Work out the finished part from the listing and answer in its coordinate system (mm). A direction names the side the tool comes from. Give positions to 0.01 mm unless a question says otherwise; leave off trailing zeros. Order: outer loops, then holes, each group sorted by start corner. A loop starts at its lowest first (then second) coordinate and runs counter-clockwise, first axis right, second up.
```python
from build123d import *

# Parameters (mm, degrees)
SKETCH1_W           = 111
SKETCH1_H           = 195
BOSS_EXTRUDE3_DEPTH = 30
SKETCH12_W          = 107
SKETCH12_H          = 191
CUT_EXTRUDE14_DEPTH = 28
SKETCH13_W          = 193
SKETCH13_H          = 26
CUT_EXTRUDE15_DEPTH = 112
CUT_EXTRUDE18_DEPTH = 28
CUT_EXTRUDE20_DEPTH = 28
FILLET1_R           = 2


with BuildPart() as part:
    # Sketch1 → Boss-Extrude3 (new body)
    with BuildSketch(Plane(origin=(0, 0, 0), x_dir=(1, 0, 0), z_dir=(0, 1, 0))):
        with Locations((55.5, 97.5)):
            Rectangle(SKETCH1_W, SKETCH1_H)
    extrude(amount=BOSS_EXTRUDE3_DEPTH)

    # Sketch12 → Cut-Extrude14 (cut)
    with BuildSketch(Plane.XZ):
        with Locations((55.5, -97.5)):
            Rectangle(SKETCH12_W, SKETCH12_H)
    extrude(amount=-CUT_EXTRUDE14_DEPTH, mode=Mode.SUBTRACT)

    # Sketch13 → Cut-Extrude15 (cut, through all)
    with BuildSketch(Plane(origin=(111, 0, 0), x_dir=(0, 0, -1), z_dir=(1, 0, 0))):
        with Locations((98.5, 13)):
            Rectangle(SKETCH13_W, SKETCH13_H)
    extrude(amount=-CUT_EXTRUDE15_DEPTH, mode=Mode.SUBTRACT)

    # Sketch14 → Cut-Extrude18 (cut)
    with BuildSketch(Plane(origin=(0, 30, 0), x_dir=(1, 0, 0), z_dir=(0, 1, 0))):
        with BuildLine():
            Line((20.333, 10), (45.333, 10))
            ThreePointArc((45.333, 10), (46.833, 11.5), (45.333, 13))
            Line((45.333, 13), (20.333, 13))
            ThreePointArc((20.333, 13), (18.833, 11.5), (20.333, 10))
        make_face()
        with BuildLine():
            Line((65.663, 10), (90.663, 10))
            ThreePointArc((90.663, 10), (92.163, 11.5), (90.663, 13))
            Line((90.663, 13), (65.663, 13))
            ThreePointArc((65.663, 13), (64.163, 11.5), (65.663, 10))
        make_face()
        with BuildLine():
            Line((45.333, 17), (20.333, 17))
            ThreePointArc((20.333, 17), (18.833, 18.5), (20.333, 20))
            Line((20.333, 20), (45.333, 20))
            ThreePointArc((45.333, 20), (46.833, 18.5), (45.333, 17))
        make_face()
        with BuildLine():
            Line((20.333, 24), (45.333, 24))
            ThreePointArc((45.333, 24), (46.833, 25.5), (45.333, 27))
            Line((45.333, 27), (20.333, 27))
            ThreePointArc((20.333, 27), (18.833, 25.5), (20.333, 24))
        make_face()
        with BuildLine():
            Line((45.333, 31), (20.333, 31))
            ThreePointArc((20.333, 31), (18.833, 32.5), (20.333, 34))
            Line((20.333, 34), (45.333, 34))
            ThreePointArc((45.333, 34), (46.833, 32.5), (45.333, 31))
        make_face()
        with BuildLine():
            Line((45.333, 38), (20.333, 38))
            ThreePointArc((20.333, 38), (18.833, 39.5), (20.333, 41))
            Line((20.333, 41), (45.333, 41))
            ThreePointArc((45.333, 41), (46.833, 39.5), (45.333, 38))
        make_face()
        with BuildLine():
            Line((65.663, 17), (90.663, 17))
            ThreePointArc((90.663, 17), (92.163, 18.5), (90.663, 20))
            Line((90.663, 20), (65.663, 20))
            ThreePointArc((65.663, 20), (64.163, 18.5), (65.663, 17))
        make_face()
        with BuildLine():
            Line((65.663, 24), (90.663, 24))
            ThreePointArc((90.663, 24), (92.163, 25.5), (90.663, 27))
            Line((90.663, 27), (65.663, 27))
            ThreePointArc((65.663, 27), (64.163, 25.5), (65.663, 24))
        make_face()
        with BuildLine():
            Line((65.663, 31), (90.663, 31))
            ThreePointArc((90.663, 31), (92.163, 32.5), (90.663, 34))
            Line((90.663, 34), (65.663, 34))
            ThreePointArc((65.663, 34), (64.163, 32.5), (65.663, 31))
        make_face()
        with BuildLine():
            Line((65.663, 38), (90.663, 38))
            ThreePointArc((90.663, 38), (92.163, 39.5), (90.663, 41))
            Line((90.663, 41), (65.663, 41))
            ThreePointArc((65.663, 41), (64.163, 39.5), (65.663, 38))
        make_face()
    extrude(amount=-CUT_EXTRUDE18_DEPTH, mode=Mode.SUBTRACT)

    # Sketch15 → Cut-Extrude20 (cut)
    with BuildSketch(Plane(origin=(0, 30, 0), x_dir=(1, 0, 0), z_dir=(0, 1, 0))):
        with BuildLine():
            ThreePointArc((6.696274737, 168.245524968), (4.712292683, 160.988985093), (4.67541183, 153.466206648))
            ThreePointArc((4.67541183, 153.466206648), (8.09565845, 150.815515518), (10.74634958, 154.235762137))
            ThreePointArc((10.74634958, 154.235762137), (10.775393211, 160.159941785), (12.337776869, 165.874458854))
            ThreePointArc((12.337776869, 165.874458854), (10.70255886, 169.880742977), (6.696274737, 168.245524968))
        make_face()
        with BuildLine():
            ThreePointArc((30.042379036, 185.905642269), (22.234806909, 183.911498962), (15.277571507, 179.845583861))
            ThreePointArc((15.277571507, 179.845583861), (14.739300825, 175.27028306), (19.314601626, 174.732012377))
            ThreePointArc((19.314601626, 174.732012377), (24.708589586, 177.884341691), (30.761848907, 179.430413423))
            ThreePointArc((30.761848907, 179.430413423), (33.639728395, 183.027762782), (30.042379036, 185.905642269))
        make_face()
        with BuildLine():
            ThreePointArc((9.491647445, 140.178899737), (15.120081319, 134.248905718), (22.173648967, 130.11474554))
            ThreePointArc((22.173648967, 130.11474554), (26.634282912, 131.979280924), (24.769747528, 136.439914869))
            ThreePointArc((24.769747528, 136.439914869), (19.370249085, 139.604610035), (15.061689013, 144.144014074))
            ThreePointArc((15.061689013, 144.144014074), (10.294111061, 144.94647769), (9.491647445, 140.178899737))
        make_face()
        with BuildLine():
            ThreePointArc((56.310614137, 175.121225777), (50.432963372, 180.790251606), (43.218248225, 184.615499013))
            ThreePointArc((43.218248225, 184.615499013), (38.682523617, 182.492393878), (40.805628753, 177.95666927))
            ThreePointArc((40.805628753, 177.95666927), (46.275147004, 175.056726572), (50.731028834, 170.75900454))
            ThreePointArc((50.731028834, 170.75900454), (55.701932104, 170.150322507), (56.310614137, 175.121225777))
        make_face()
        with BuildLine():
            ThreePointArc((59.586594576, 144.047302408), (62.128106042, 151.638527757), (62.527114252, 159.633949903))
            ThreePointArc((62.527114252, 159.633949903), (58.568776784, 162.958953376), (55.24377331, 159.000615908))
            ThreePointArc((55.24377331, 159.000615908), (54.944008323, 152.99385325), (53.034633698, 147.290753636))
            ThreePointArc((53.034633698, 147.290753636), (54.688888523, 142.393047582), (59.586594576, 144.047302408))
        make_face()
        with BuildLine():
            ThreePointArc((35.768008384, 128.065909487), (43.426937588, 129.793958929), (50.34619431, 133.504651297))
            ThreePointArc((50.34619431, 133.504651297), (51.101165333, 138.243900564), (46.361916066, 138.998871587))
            ThreePointArc((46.361916066, 138.998871587), (41.05466641, 136.152674144), (35.180068745, 134.827215331))
            ThreePointArc((35.180068745, 134.827215331), (32.093385643, 131.15259259), (35.768008384, 128.065909487))
        make_face()
        with BuildLine():
            ThreePointArc((16.441661235, 152.073186373), (17.981802443, 148.454567611), (20.289670934, 145.270202728))
            ThreePointArc((20.289670934, 145.270202728), (24.525226929, 145.075748549), (24.719681108, 149.311304544))
            ThreePointArc((24.719681108, 149.311304544), (23.201014452, 151.406739699), (22.187542017, 153.787930688))
            ThreePointArc((22.187542017, 153.787930688), (18.457229469, 155.803498921), (16.441661235, 152.073186373))
        make_face()
        with BuildLine():
            ThreePointArc((29.27435513, 140.205739876), (33.244380925, 139.745216), (37.21440672, 140.205739876))
            ThreePointArc((37.21440672, 140.205739876), (39.303217461, 143.579049176), (35.929908161, 145.667859918))
            ThreePointArc((35.929908161, 145.667859918), (33.244380925, 145.356338161), (30.558853689, 145.667859918))
            ThreePointArc((30.558853689, 145.667859918), (27.185544389, 143.579049176), (29.27435513, 140.205739876))
        make_face()
        with BuildLine():
            ThreePointArc((46.62439771, 146.108244738), (48.343223739, 148.626148349), (49.593608613, 151.406569032))
            ThreePointArc((49.593608613, 151.406569032), (47.885475932, 154.933944656), (44.358100308, 153.225811975))
            ThreePointArc((44.358100308, 153.225811975), (43.508125809, 151.335764577), (42.339718927, 149.624168488))
            ThreePointArc((42.339718927, 149.624168488), (42.724096443, 145.723867222), (46.62439771, 146.108244738))
        make_face()
        with BuildLine():
            ThreePointArc((49.972810261, 162.900447104), (48.635358132, 165.848165567), (46.783719502, 168.503209204))
            ThreePointArc((46.783719502, 168.503209204), (42.312959082, 168.883687171), (41.932481115, 164.412926751))
            ThreePointArc((41.932481115, 164.412926751), (43.120664854, 162.709203559), (43.978898661, 160.817672951))
            ThreePointArc((43.978898661, 160.817672951), (48.017241537, 158.862104227), (49.972810261, 162.900447104))
        make_face()
        with BuildLine():
            ThreePointArc((20.111654536, 168.296978183), (17.884918862, 164.974641199), (16.482333682, 161.229106577))
            ThreePointArc((16.482333682, 161.229106577), (18.47726406, 157.924889924), (21.781480713, 159.919820302))
            ThreePointArc((21.781480713, 159.919820302), (22.740653165, 162.48124308), (24.263429498, 164.753257755))
            ThreePointArc((24.263429498, 164.753257755), (23.959402231, 168.601005449), (20.111654536, 168.296978183))
        make_face()
        with BuildLine():
            ThreePointArc((36.492341368, 174.366325724), (33.369121981, 174.668500564), (30.241929234, 174.410674085))
            ThreePointArc((30.241929234, 174.410674085), (27.762102428, 170.891007932), (31.281768581, 168.411181126))
            ThreePointArc((31.281768581, 168.411181126), (33.3259204, 168.579714539), (35.367474954, 168.382191937))
            ThreePointArc((35.367474954, 168.382191937), (38.921975054, 170.811825623), (36.492341368, 174.366325724))
        make_face()
    extrude(amount=-CUT_EXTRUDE20_DEPTH, mode=Mode.SUBTRACT)

    # Fillet1
    fillet1_edges = [part.edges().sort_by_distance(p)[0] for p in [
        (55.5, 30, 0),
    ]]
    fillet(fillet1_edges, radius=FILLET1_R)


solid = part.part
```
1. Given P1, Ø0.6, axis at x = 33, y = 29, coming from the +Z side; P2, Ø1.6, axis at x = 29.5, y = 29, coming from the +Z side; P3, Ø4, axis at x = 58, y = 12, coming from the -Z side, each flat-ended and moving along its own axis, determine where each tip first touches the part or whether it passes through.
Findings below:
P1: stops at z = -0.13
P2: stops at z = -0.01
P3: stops at z = -2
2. The part is cut by section B-B (z = -115.5). Write down the section's boundary in (x, y), then the cut area to 3 significant figures.
Findings below:
outline: (0, 26) - (2, 26) - (2, 28) - (109, 28) - (109, 26) - (111, 26) - (111, 30) - (0, 30) - close
area: 230 mm2
3. The mould has two halves that part along Z. Classify faces 1 (the face through (27.75, 29.01, -170.96)), 2 (the face through (111, 27, -97)): pulls with the +Z half, pulls with the -Z half, needs draft (parallel to the pull), parting line crosses it, or undercut.
Findings below:
face 1: undercut
face 2: needs draft
4. The part is cut by section C-C (y = 22.5). Write down the section's boundary in (x, z).
Findings below:
outline: (0, -2) - (111, -2) - (111, 0) - (0, 0) - close
5. The part is cut by section A-A (x = 68.5). State how many separate pieces and enclosed holes the cut face has, then the cut area to 3 significant figures.
Findings below:
separate pieces: 6
enclosed holes: 0
area: 419 mm2
6. Straight lines are drawn through the part: probe 1 along X at (y, z) = (27.5, -87); probe 2 along Z at (x, y) = (51.5, 27.25); probe 3 along Y at (x, z) = (37.5, -181.5). For each, find the intervals that lie inside material, in ascending order.
Findings below:
probe 1: x = 0 to 2, 109 to 111
probe 2: z = -195 to -193, -2 to 0
probe 3: y = 28 to 30
7. Which of the six approach directions +Z, -Z, +X, -X, +Y, -Y give full straight-line access (tool end or side, diameter ignored) to faces 3 (the face through (55, 30, -100)), 4 (the face through (46.2, 29.01, -175.11))?
Findings below:
face 3: +Z, -Z, +X, -X, +Y
face 4: +Y, -Y
